from build123d import *

# Parameters (mm, degrees)
BOSS_EXTRUDE1_DEPTH      = 3.175
BOSS_EXTRUDE2_DEPTH      = 3.175
BOSS_EXTRUDE2_DEPTH_BACK = 34.925
SKETCH2_W                = 31.75
SKETCH2_H                = 3.175
CUT_EXTRUDE1_DEPTH       = 111.671398355
F_4_CLEARANCE_HOLE1_D    = 2.9464


with BuildPart() as part:
    # Sketch1 → Boss-Extrude1 (new body)
    with BuildSketch(Plane(origin=(0, 0, -14.15699402), x_dir=(-1, 0, 0), z_dir=(0, 0, -1))):
        with BuildLine():
            Line((-49.172312317, -34.502108483), (-53.141062317, -27.628031841))
            ThreePointArc((-53.141062317, -27.628031841), (-55.063803638, -24.012221257), (-56.72992661, -20.271224785))
            ThreePointArc((-56.72992661, -20.271224785), (-54.976138042, -16.13776671), (-50.842679967, -17.891555277))
            ThreePointArc((-50.842679967, -17.891555277), (-49.356678398, -21.228119699), (-47.641801003, -24.453031841))
            Line((-47.641801003, -24.453031841), (-43.673051003, -31.327108483))
            ThreePointArc((-43.673051003, -31.327108483), (-16.68272836, -52.037511462), (17.046778195, -47.596937682))
            Line((17.046778195, -47.596937682), (23.920854837, -43.628187682))
            Line((23.920854837, -43.628187682), (30.79493148, -39.659437682))
            ThreePointArc((30.79493148, -39.659437682), (51.505334458, -12.669115038), (47.064760678, 21.060391517))
            Line((47.064760678, 21.060391517), (43.096010678, 27.934468159))
            ThreePointArc((43.096010678, 27.934468159), (41.160593535, 31.032051618), (39.01404477, 33.987248938))
            ThreePointArc((39.01404477, 33.987248938), (39.561948355, 38.44382292), (44.018522337, 37.895919335))
            ThreePointArc((44.018522337, 37.895919335), (46.425258832, 34.58251628), (48.595271992, 31.109468159))
            Line((48.595271992, 31.109468159), (52.564021992, 24.235391517))
            ThreePointArc((52.564021992, 24.235391517), (57.638963455, -14.312615975), (33.96993148, -45.158698996))
            Line((33.96993148, -45.158698996), (27.095854837, -49.127448996))
            Line((27.095854837, -49.127448996), (20.221778195, -53.096198996))
            ThreePointArc((20.221778195, -53.096198996), (-18.326229296, -58.171140459), (-49.172312317, -34.502108483))
        make_face()
    extrude(amount=BOSS_EXTRUDE1_DEPTH)

    # Sketch2 → Boss-Extrude2 (add, two sides: drawn at the far end of the back side and taken through both)
    with BuildSketch(Plane(origin=(8.682443514, -58.42, 0), x_dir=(-1, 0, 0), z_dir=(0, 1, 0)).offset(-BOSS_EXTRUDE2_DEPTH_BACK)):
        with Locations((1.098025871, -15.74449402)):
            Rectangle(SKETCH2_W, SKETCH2_H)
    extrude(amount=BOSS_EXTRUDE2_DEPTH + BOSS_EXTRUDE2_DEPTH_BACK)

    # Sketch3 → Cut-Extrude1 (cut, through all)
    with BuildSketch(Plane(origin=(0, 0, -17.33199402), x_dir=(-1, 0, 0), z_dir=(0, 0, -1))):
        with BuildLine():
            Line((-20.534417629, -67.17), (-20.534417629, -63.17))
            ThreePointArc((-20.534417629, -63.17), (-19.084417629, -61.72), (-17.634417629, -63.17))
            Line((-17.634417629, -63.17), (-17.634417629, -67.17))
            ThreePointArc((-17.634417629, -67.17), (-19.084417629, -68.62), (-20.534417629, -67.17))
        make_face()
        with BuildLine():
            Line((2.465582371, -67.17), (2.465582371, -63.17))
            ThreePointArc((2.465582371, -63.17), (3.915582371, -61.72), (5.365582371, -63.17))
            Line((5.365582371, -63.17), (5.365582371, -67.17))
            ThreePointArc((5.365582371, -67.17), (3.915582371, -68.62), (2.465582371, -67.17))
        make_face()
        with BuildLine():
            Line((-20.534417629, -90.17), (-20.534417629, -86.17))
            ThreePointArc((-20.534417629, -86.17), (-19.084417629, -84.72), (-17.634417629, -86.17))
            Line((-17.634417629, -86.17), (-17.634417629, -90.17))
            ThreePointArc((-17.634417629, -90.17), (-19.084417629, -91.62), (-20.534417629, -90.17))
        make_face()
        with BuildLine():
            Line((2.465582371, -90.17), (2.465582371, -86.17))
            ThreePointArc((2.465582371, -86.17), (3.915582371, -84.72), (5.365582371, -86.17))
            Line((5.365582371, -86.17), (5.365582371, -90.17))
            ThreePointArc((5.365582371, -90.17), (3.915582371, -91.62), (2.465582371, -90.17))
        make_face()
        with BuildLine():
            Line((-18.584417642, -78.67), (-18.584417642, -74.67))
            ThreePointArc((-18.584417642, -74.67), (-7.584417642, -63.67), (3.415582358, -74.67))
            Line((3.415582358, -74.67), (3.415582358, -78.67))
            ThreePointArc((3.415582358, -78.67), (-7.584417642, -89.67), (-18.584417642, -78.67))
        make_face()
    extrude(amount=-CUT_EXTRUDE1_DEPTH, mode=Mode.SUBTRACT)

    # #4 Clearance Hole1 (through all)
    with Locations(Plane(origin=(0, 0, -17.33199402), x_dir=(-1, 0, 0), z_dir=(0, 0, -1))):
        with Locations((-53.56643166, -20.541270527), (-47.21643166, -31.539793155), (42.670641335, 35.021229473), (49.020641335, 24.022706845)):
            Hole(F_4_CLEARANCE_HOLE1_D / 2)


solid = part.part
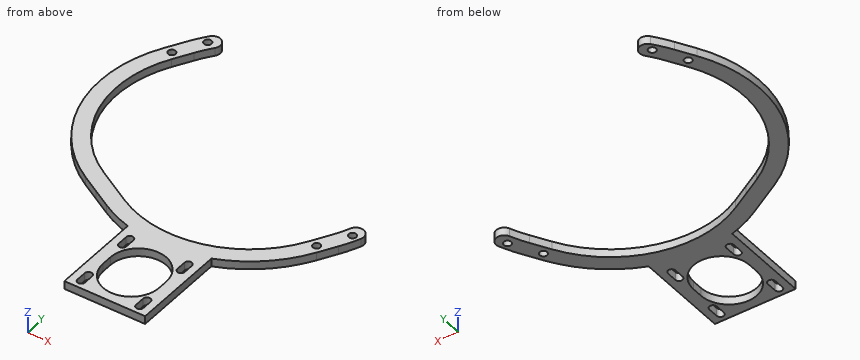
Source: CAD feature listing. Evaluate the final solid. Frame: model axes, mm. Give positions to 0.01 mm unless a question says otherwise; leave off trailing zeros. Order: outer loops, then holes, each group sorted by start corner. A loop starts at its lowest first (then second) coordinate and runs counter-clockwise, first axis right, second up. Notation, with made-up numbers: (72.5, 65) -> (92.5, 65) arc R24 ccw to (92.5, 80) -> close; hole circle Ø2 at (55.5, 2.5). An arc over 180 degrees is marked (long way). Use a Markdown table: item, result.
1) Section query A-A, the plane y = -65.5. Return the cut outline in (x, z), then the cut area to 3 significant figures.
Answer list:
| item | result |
|---|---|
| outline | (-8.29, -17.33) -> (-5.37, -17.33) -> (-5.37, -14.16) -> (-8.29, -14.16) -> close; (-2.47, -17.33) -> (1.51, -17.33) -> (1.51, -14.16) -> (-2.47, -14.16) -> close; (13.66, -17.33) -> (17.63, -17.33) -> (17.63, -14.16) -> (13.66, -14.16) -> close; (20.53, -17.33) -> (23.46, -17.33) -> (23.46, -14.16) -> (20.53, -14.16) -> close |
| area | 43.8 mm² |
2) Section query B-B, the plane x = 11. Return the cut outline in (y, z) (3 decimals), then the cut area to 3 significant figures.
Answer list:
| item | result |
|---|---|
| outline | (-93.345, -17.332) -> (-89.126, -17.332) -> (-89.126, -14.157) -> (-93.345, -14.157) -> close; (-64.214, -17.332) -> (-53.169, -17.332) -> (-53.169, -14.157) -> (-64.214, -14.157) -> close |
| area | 48.5 mm² |
3) Ray query, line 1 along X through (y, z) = (-88, -14.7); line 2 along X through (y, z) = (-58.5, -15.45); line 3 along X through (y, z) = (-46, -14.75). Return the intervals inside material, ascending. Write a range as [from, to].
Answer list:
| item | result |
|---|---|
| line 1 | [-8.29, -5.37], [-2.47, 1.76], [13.41, 17.63], [20.53, 23.46] |
| line 2 | [-8.29, 23.46] |
| line 3 | [-32.51, -19.81], [29.96, 40.1] |
4) Contact query for flat-ended pins moving along their axis: P1, Ø2.5, axis at x = 53.57, y = -20.54, coming from the -Z side; P2, Ø1.6, axis at y = -65.5, z = -16.5, coming from the +X side; P3, Ø4, axis at x = 47.22, y = -31.54, coming from the +Z side; P4, Ø1, axis at y = -87.5, z = -15.5, coming from the -X side. Output: stop coordinate, or through.
Answer list:
| item | result |
|---|---|
| P1 | through |
| P2 | x = 23.46 |
| P3 | z = -14.16 |
| P4 | x = -8.29 |
5) Section query C-C, the plane z = -16.5. Count the separate pieces of the cut face and the enclosed holes in it, then the cut area to 3 significant figures.
Answer list:
| item | result |
|---|---|
| separate pieces | 1 |
| enclosed holes | 9 |
| area | 1,800 mm² |
